Could you check a few things on this model? Use its own coordinates, in mm. Face numbers are marked on the shaded views. A direction names the side the tool comes from. Coordinates: 2 decimals unless noted, no trailing zeros. Loops run counter-clockwise (first coordinate to the right, second up) from the corner with the lowest first, then second, coordinate; pieces in that order, holes last. Notation, with made-up numbers: (51.25, -8.75) -> (82.25, -8.75) arc R5 cw to (82.25, -0.75) -> close; hole circle Ø8 at (-29.75, -16.5). An arc over 180 degrees is marked (long way). One line per question, with ' | ' between items.
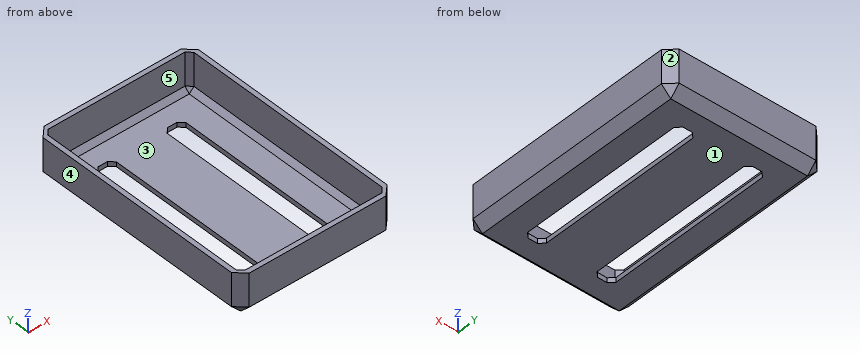
from build123d import *

# Parameters (mm, degrees)
F0_W     = 62
F0_H     = 94
F0_W_2   = 8
F0_H_2   = 74
F1_DEPTH = 2
F2_DEPTH = 18
F3_SIZE  = 2
F4_SIZE  = 4


with BuildPart() as f1:
    # F0 (on Top) → F1 (new body)
    with BuildSketch(Plane.XY):
        Polygon((-33, -44), (-33, -49), (33, -49), (33, 49), (-33, 49), (-33, 44), align=None)
        Rectangle(F0_W, F0_H, mode=Mode.SUBTRACT)
        Rectangle(F0_W, F0_H)
        with Locations((-14.75, 0)):
            Rectangle(F0_W_2, F0_H_2, mode=Mode.SUBTRACT)
        with Locations((14.75, 0)):
            Rectangle(F0_W_2, F0_H_2, mode=Mode.SUBTRACT)
    extrude(amount=F1_DEPTH)

    # F0 (on Top) → F2 (join)
    with BuildSketch(Plane.XY):
        Polygon((-33, -44), (-33, -49), (33, -49), (33, 49), (-33, 49), (-33, 44), align=None)
        Rectangle(F0_W, F0_H, mode=Mode.SUBTRACT)
    extrude(amount=F2_DEPTH)

    # F3
    f3_edges = [f1.edges().sort_by_distance(p)[0] for p in [
        (31, 47, 10),
        (-31, 47, 10),
        (-31, -47, 10),
        (31, -47, 10),
        (-18.75, 37, 1),
        (10.75, 37, 1),
        (-10.75, 37, 1),
        (18.75, 37, 1),
        (-10.75, -37, 1),
        (18.75, -37, 1),
        (10.75, -37, 1),
        (-18.75, -37, 1),
        (-31, 0, 2),
        (0, 47, 2),
        (31, 0, 2),
        (0, -47, 2),
    ]]
    chamfer(f3_edges, length=F3_SIZE)

    # F4
    f4_edges = [f1.edges().sort_by_distance(p)[0] for p in [
        (-33, 49, 9),
        (33, 49, 9),
        (33, -49, 9),
        (-33, -49, 9),
        (-33, 0, 0),
        (33, 0, 0),
        (0, -49, 0),
        (0, 49, 0),
    ]]
    chamfer(f4_edges, length=F4_SIZE)


solid = f1.part
1) If we section it at D-D on x = 27: Please give me the cut outline in (y, z).
Data:
outline: (-49, 4) -> (-45, 0) -> (45, 0) -> (49, 4) -> (49, 18) -> (47, 18) -> (47, 4) -> (45, 2) -> (-45, 2) -> (-47, 4) -> (-47, 18) -> (-49, 18) -> close
2) We'd pull the mould along Y, two halves only. Please class the marked faces 1, 2 and 3: pulls with the +Y half, pulls with the -Y half, needs draft (parallel to the pull), parting line crosses it, or undercut.
Data:
face 1: needs draft | face 2: pulls with the +Y half | face 3: undercut
3) I need wall thicknesses on line 1 along Y through (x, z) = (1.5, 15.5); line 2 along X through (y, z) = (40, 6.5); line 3 along Z through (x, y) = (0, 9). Which ranges of each line are inside material? Lowest first, please. Write a range as from..to.
Data:
line 1: -49..-47, 47..49 | line 2: -33..-31, 31..33 | line 3: 0..2
4) I'm going to push flat-ended pins straight in: pin 1 Ø0.6 at (y, z) = (-16.5, 1) entering from +X; pin 2 Ø1.6 at (y, z) = (-0.5, 1) entering from -X; pin 3 Ø17.5 at (x, y) = (9, -7.5) entering from +Z; pin 4 Ø12 at (x, y) = (12.5, 25.5) entering from -Z. Where does each tip first touch, or does it pass through?
Data:
pin 1: x = 30.3 | pin 2: x = -30.8 | pin 3: z = 2 | pin 4: z = 0
5) If we section it at A-A on y = 14: Please give me the cut outline in (x, z).
Data:
outline: (-33, 4) -> (-29, 0) -> (-18.75, 0) -> (-18.75, 2) -> (-29, 2) -> (-31, 4) -> (-31, 18) -> (-33, 18) -> close; (-10.75, 0) -> (10.75, 0) -> (10.75, 2) -> (-10.75, 2) -> close; (18.75, 0) -> (29, 0) -> (33, 4) -> (33, 18) -> (31, 18) -> (31, 4) -> (29, 2) -> (18.75, 2) -> close
6) If we section it at B-B on z = 15.25: Please give me the cut outline in (x, y).
Data:
outline: (-33, -45) -> (-29, -49) -> (29, -49) -> (33, -45) -> (33, 45) -> (29, 49) -> (-29, 49) -> (-33, 45) -> close; hole (-31, -45) -> (-29, -47) -> (29, -47) -> (31, -45) -> (31, 45) -> (29, 47) -> (-29, 47) -> (-31, 45) -> close
7) If we section it at C-C on x = 14: Please give me the cut outline in (y, z), and give its area (3 significant figures).
Data:
outline: (-49, 4) -> (-45, 0) -> (-37, 0) -> (-37, 2) -> (-45, 2) -> (-47, 4) -> (-47, 18) -> (-49, 18) -> close; (37, 0) -> (45, 0) -> (49, 4) -> (49, 18) -> (47, 18) -> (47, 4) -> (45, 2) -> (37, 2) -> close | area: 100 mm²
8) On a 3-axis mill with a long thin cutter (end or side, diameter ignored), from which of +Z, -Z, +X, -X, +Y, -Y can I reach the whole of each face in a straight line? I mean the marked faces 4 and 5. Say none if no direction works.
Data:
face 4: +Z, -Z, -X, +Y, -Y | face 5: +Z
